```python
from build123d import *

# Parameters (mm, degrees)
SKETCH_1_W          = 70
SKETCH_1_H          = 30
EXTRUDE_1_DEPTH     = 4
SKETCH_2_W          = 12
SKETCH_2_H          = 20
EXTRUDE_2_DEPTH     = 20
SKETCH_7_R          = 1.5
CUT_EXTRUDE_2_DEPTH = 12
SKETCH_11_R         = 1.55
CUT_EXTRUDE_4_DEPTH = 50
FILLET_1_R          = 10
FILLET_2_R          = 10


with BuildPart() as part:
    # 草图1 → 凸台-拉伸1 (new body)
    with BuildSketch(Plane(origin=(0, 0, 0), x_dir=(1, 0, 0), z_dir=(0, 1, 0))):
        with Locations((35, -15)):
            Rectangle(SKETCH_1_W, SKETCH_1_H)
    extrude(amount=EXTRUDE_1_DEPTH)

    # 草图2 → 凸台-拉伸2 (add)
    with BuildSketch(Plane(origin=(0, 4, 0), x_dir=(1, 0, 0), z_dir=(0, 1, 0))):
        with Locations((10.5, -15)):
            Rectangle(SKETCH_2_W, SKETCH_2_H)
    extrude(amount=EXTRUDE_2_DEPTH)

    # 草图7 → 切除-拉伸2 (cut)
    with BuildSketch(Plane(origin=(16.5, 0, 0), x_dir=(0, 0, -1), z_dir=(1, 0, 0))):
        with Locations((-15, 14)):
            Circle(SKETCH_7_R)
    extrude(amount=-CUT_EXTRUDE_2_DEPTH, mode=Mode.SUBTRACT)

    # 草图11 → 切除-拉伸4 (cut)
    with BuildSketch(Plane(origin=(0, 4, 0), x_dir=(1, 0, 0), z_dir=(0, 1, 0))):
        with Locations(Location((55, -15, 0), (0, 0, 270))):
            Circle(SKETCH_11_R)
        with Locations(Location((50, -23.660254038, 0), (0, 0, 270))):
            Circle(SKETCH_11_R)
        with Locations(Location((46.339745962, -20, 0), (0, 0, 270))):
            Circle(SKETCH_11_R)
        with Locations(Location((46.339745962, -10, 0), (0, 0, 270))):
            Circle(SKETCH_11_R)
        with Locations(Location((50, -6.339745962, 0), (0, 0, 270))):
            Circle(SKETCH_11_R)
        with Locations(Location((45, -15, 0), (0, 0, 270))):
            Circle(SKETCH_11_R)
        with Locations(Location((55, -5, 0), (0, 0, 270))):
            Circle(SKETCH_11_R)
        with Locations(Location((55, -25, 0), (0, 0, 270))):
            Circle(SKETCH_11_R)
    extrude(amount=-CUT_EXTRUDE_4_DEPTH, mode=Mode.SUBTRACT)

    # 圆角1
    fillet_1_edges = [part.edges().sort_by_distance(p)[0] for p in [
        (70, 2, 30),
    ]]
    fillet(fillet_1_edges, radius=FILLET_1_R)

    # 圆角2
    fillet_2_edges = [part.edges().sort_by_distance(p)[0] for p in [
        (70, 2, 0),
    ]]
    fillet(fillet_2_edges, radius=FILLET_2_R)


solid = part.part
```
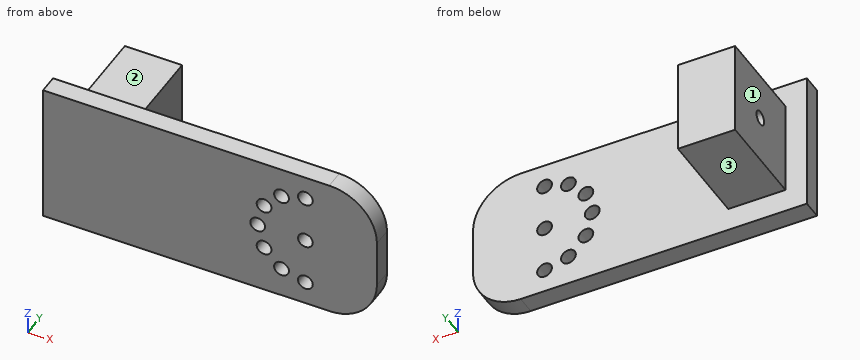
The listing builds one solid part. Answer for the finished solid, in the listing's coordinates (mm). Face numbers are marked on the shaded views. A direction names the side the tool comes from. Give positions to 0.01 mm unless a question says otherwise; leave off trailing zeros. Write each loop counter-clockwise with the first axis right and the second up, starting at its lowest first coordinate (ties: lowest second). Pieces come first, ordered by that corner, then holes. Notation, with made-up numbers: (-24, 50.5) - (11, 50.5) arc R13 ccw to (11, 73.5) - close; hole circle Ø4 at (13, -7.75). An arc over 180 degrees is marked (long way). Use one line per item in the form item = value. Start each with the question number.
1) Flat-ended cylindrical pins translate along their axes: pin 1 Ø6 at (x, y) = (10.5, 11.5) entering from -Z; pin 2 Ø2 at (x, z) = (13.5, 14) entering from -Y; pin 3 Ø9.5 at (x, y) = (11, 12) entering from +Z; pin 4 Ø1.5 at (y, z) = (21.5, 7) entering from +X. Find the tip coordinate at first contact, or state that the pin passes through.
2) Find section B-B on x = 55. Determine the outline of the cut face in (y, z).
3) Find section A-A on x = 6. Determine the outline of the cut face in (y, z), plus the area to 3 significant figures.
4) Find section C-C on z = 15. Determine the outline of the cut face in (x, y), plus the area to 3 significant figures.
5) A tool of negligible diameter and unlimited length cuts with its end or side. For the marked faces 1, 2 and 3, from which of +Z, -Z, +X, -X, +Y, -Y can it reach the whole face along a straight path? Write none if from no direction.
6) Consider line 1 along Y through (x, z) = (64, 17); line 2 along X through (y, z) = (18.5, 14.25); line 3 along X through (y, z) = (1.4, 25). Determine where each line is inside the solid, lowest interval first. Write a range as from..to.
7) Find section D-D on y = 21.5. Determine the outline of the cut face in (x, z).
Geometry results:
q1.pin_1 = 5
q1.pin_2 = 0
q1.pin_3 = 25
q1.pin_4 = 16.5
q2.outline = (0, 0) - (4, 0) - (4, 3.45) - (0, 3.45) - close; (0, 6.55) - (4, 6.55) - (4, 13.45) - (0, 13.45) - close; (0, 16.55) - (4, 16.55) - (4, 23.45) - (0, 23.45) - close; (0, 26.55) - (4, 26.55) - (4, 30) - (0, 30) - close
q3.outline = (0, 0) - (4, 0) - (4, 5) - (24, 5) - (24, 25) - (4, 25) - (4, 30) - (0, 30) - close; hole circle Ø3 at (14, 15)
q3.area = 513 mm2
q4.outline = (0, 0) - (43.45, 0) - (43.45, 4) - (16.5, 4) - (16.5, 12.5) - (4.5, 12.5) - (4.5, 4) - (0, 4) - close; (4.5, 15.5) - (16.5, 15.5) - (16.5, 24) - (4.5, 24) - close; (46.55, 0) - (53.45, 0) - (53.45, 4) - (46.55, 4) - close; (56.55, 0) - (70, 0) - (70, 4) - (56.55, 4) - close
q4.area = 459 mm2
q5.face_1 = +Z, -Z, -X, +Y
q5.face_2 = +Z, +X, -X, +Y
q5.face_3 = -Z, +X, -X, +Y
q6.line_1 = 0..4
q6.line_2 = 4.5..16.5
q6.line_3 = 0..49.22, 50.78..53.45, 56.55..68.66
q7.outline = (4.5, 5) - (16.5, 5) - (16.5, 25) - (4.5, 25) - close
